For this review, take the finished solid that the model builds, in its own axes (mm). A direction names the side the tool comes from. Give positions to 0.01 mm unless a question says otherwise; leave off trailing zeros. Order: outer loops, then holes, each group sorted by start corner. A loop starts at its lowest first (then second) coordinate and runs counter-clockwise, first axis right, second up.
from build123d import *

# Parameters (mm, degrees)
SKETCH_1_R          = 1.6
SKETCH_1_R_2        = 30
SKETCH_1_R_3        = 2.1
EXTRUDE_1_DEPTH     = 2.5
SKETCH_2_W          = 20
SKETCH_2_H          = 5
EXTRUDE_2_DEPTH     = 5
CUT_EXTRUDE_1_DEPTH = 97.176920308
FILLET_1_R          = 5


with BuildPart() as part:
    # 草图1 → 凸台-拉伸1 (new, symmetric)
    with BuildSketch(Plane(origin=(0, 0, 0), x_dir=(1, 0, 0), z_dir=(0, 1, 0))):
        with BuildLine():
            Line((-60, 0), (-60, -70))
            Line((-60, -70), (60, -70))
            Line((60, -70), (60, 0))
            ThreePointArc((60, 0), (42.426406871, 42.426406871), (0, 60))
            ThreePointArc((0, 60), (-42.426406871, 42.426406871), (-60, 0))
        make_face()
        with Locations(Location((-37.5, 0, 0), (0, 0, 270))):
            Circle(SKETCH_1_R, mode=Mode.SUBTRACT)
        with Locations(Location((-40, -57.62, 0), (0, 0, 270))):
            Circle(SKETCH_1_R, mode=Mode.SUBTRACT)
        with Locations(Location((40, -57.62, 0), (0, 0, 270))):
            Circle(SKETCH_1_R, mode=Mode.SUBTRACT)
        with Locations(Location((0, 0, 0), (0, 0, 270))):
            Circle(SKETCH_1_R_2, mode=Mode.SUBTRACT)
        with Locations(Location((-28.726666617, 24.104535363, 0), (0, 0, 270))):
            Circle(SKETCH_1_R, mode=Mode.SUBTRACT)
        with Locations(Location((-6.511806663, 36.930290738, 0), (0, 0, 270))):
            Circle(SKETCH_1_R, mode=Mode.SUBTRACT)
        with Locations(Location((18.75, 32.475952642, 0), (0, 0, 270))):
            Circle(SKETCH_1_R, mode=Mode.SUBTRACT)
        with Locations(Location((35.238473279, 12.825755375, 0), (0, 0, 270))):
            Circle(SKETCH_1_R, mode=Mode.SUBTRACT)
        with Locations(Location((35.238473279, -12.825755375, 0), (0, 0, 270))):
            Circle(SKETCH_1_R, mode=Mode.SUBTRACT)
        with Locations(Location((18.75, -32.475952642, 0), (0, 0, 270))):
            Circle(SKETCH_1_R, mode=Mode.SUBTRACT)
        with Locations(Location((-6.511806663, -36.930290738, 0), (0, 0, 270))):
            Circle(SKETCH_1_R, mode=Mode.SUBTRACT)
        with Locations(Location((-28.726666617, -24.104535363, 0), (0, 0, 270))):
            Circle(SKETCH_1_R, mode=Mode.SUBTRACT)
        with Locations(Location((-11, -65, 0), (0, 0, 270))):
            Circle(SKETCH_1_R_3, mode=Mode.SUBTRACT)
        with Locations(Location((11, -65, 0), (0, 0, 90))):
            Circle(SKETCH_1_R_3, mode=Mode.SUBTRACT)
        with Locations(Location((40, -47.62, 0), (0, 0, 270))):
            Circle(SKETCH_1_R_3, mode=Mode.SUBTRACT)
        with Locations(Location((40, -37.62, 0), (0, 0, 270))):
            Circle(SKETCH_1_R_3, mode=Mode.SUBTRACT)
        with Locations(Location((40, -27.62, 0), (0, 0, 270))):
            Circle(SKETCH_1_R_3, mode=Mode.SUBTRACT)
        with Locations(Location((0, -54, 0), (0, 0, 270))):
            Circle(SKETCH_1_R, mode=Mode.SUBTRACT)
        with Locations(Location((8.488193337, 40, 0), (0, 0, 270))):
            Circle(SKETCH_1_R, mode=Mode.SUBTRACT)
        with Locations(Location((-1.511806663, 40.862744239, 0), (0, 0, 270))):
            Circle(SKETCH_1_R, mode=Mode.SUBTRACT)
        with Locations(Location((-11.420717282, 39.263426275, 0), (0, 0, 270))):
            Circle(SKETCH_1_R, mode=Mode.SUBTRACT)
    extrude(amount=EXTRUDE_1_DEPTH, both=True)

    # 草图2 → 凸台-拉伸2 (add)
    with BuildSketch(Plane.XY.offset(70)):
        with Locations((40, 0)):
            Rectangle(SKETCH_2_W, SKETCH_2_H)
        with Locations((-40, 0)):
            Rectangle(SKETCH_2_W, SKETCH_2_H)
    extrude(amount=EXTRUDE_2_DEPTH)

    # 草图3 → 切除-拉伸1 (cut, through all)
    with BuildSketch(Plane(origin=(0, 2.5, 0), x_dir=(1, 0, 0), z_dir=(0, 1, 0))):
        with BuildLine():
            ThreePointArc((41.406951107, -17.62), (0, 45), (-41.406951107, -17.62))
            Line((-41.406951107, -17.62), (-60, -70))
            Line((-60, -70), (-60, 0))
            ThreePointArc((-60, 0), (0, 60), (60, 0))
            Line((60, 0), (60, -70))
            Line((60, -70), (41.406951107, -17.62))
        make_face()
    extrude(amount=-CUT_EXTRUDE_1_DEPTH, mode=Mode.SUBTRACT)

    # 圆角1
    fillet_1_edges = [part.edges().sort_by_distance(p)[0] for p in [
        (60, 0, 70),
        (-60, 0, 70),
    ]]
    fillet(fillet_1_edges, radius=FILLET_1_R)


solid = part.part
1) We need section A-A on z = 0. Give the boundary of the cut face in (x, y), then the cut area to 3 significant figures.
Answer sheet:
outline: (-45, -2.5) - (-39.1, -2.5) - (-39.1, 2.5) - (-45, 2.5) - close; (-35.9, -2.5) - (-30, -2.5) - (-30, 2.5) - (-35.9, 2.5) - close; (30, -2.5) - (45, -2.5) - (45, 2.5) - (30, 2.5) - close
area: 134 mm2
2) We need section D-D on z = 43. Give the boundary of the cut face in (x, y).
Answer sheet:
outline: (-50.42, -2.5) - (50.42, -2.5) - (50.42, 2.5) - (-50.42, 2.5) - close
3) Draft analysis for pull direction X (two halves, no side actions). For faces 4 (the face through (1.243, 0.035, -44.983)), 5 (the face through (-1, -2.5, 41)), 6 (the face through (-1.031, -0.035, -39.337)), state which applies: +X half, -X half, draft (parallel to the pull), parting line (faces both ways), or undercut.
Answer sheet:
face 4: parting line
face 5: draft
face 6: undercut
4) To check wall thickness, follow line 1 (X direction, y = -1.15, z = 0); line 2 (X direction, y = 1.45, z = -40); line 3 (X direction, y = 1.15, z = 36). State the ranges of each line that lie inside material, in increasing order.
Answer sheet:
line 1: x = -45 to -39.1, -35.9 to -30, 30 to 45
line 2: x = -20.62 to -12.84, -10 to -2.86, -0.16 to 6.89, 10.09 to 20.62
line 3: x = -47.93 to -7.81, -5.21 to 38.66, 41.34 to 47.93
5) We need section C-C on z = 27.62. Give the boundary of the cut face in (x, y), then the cut area to 3 significant figures.
Answer sheet:
outline: (-44.96, -2.5) - (-11.71, -2.5) - (-11.71, 2.5) - (-44.96, 2.5) - close; (11.71, -2.5) - (37.9, -2.5) - (37.9, 2.5) - (11.71, 2.5) - close; (42.1, -2.5) - (44.96, -2.5) - (44.96, 2.5) - (42.1, 2.5) - close
area: 311 mm2
6) Clearance check with flat-ended pins moving along their axes: pin 1 (1.5 mm diameter, centred on y = 0, z = 72, fed in from -X); pin 2 (4 mm diameter, centred on x = -28.73, z = 24.1, fed in from -Y); pin 3 (1 mm diameter, centred on y = -0.5, z = 37, fed in from -X); pin 4 (2 mm diameter, centred on y = 0.5, z = 9, fed in from +X). State where each tip first meets the part, or that it passes through.
Answer sheet:
pin 1: stops at x = -50
pin 2: stops at y = -2.5
pin 3: stops at x = -48.46
pin 4: stops at x = 44.28
7) Tool access review of faces 1 (the face through (-50, 0, 72)), 2 (the face through (-30, 0, 72)), 3 (the face through (49.63, 0.04, 40.79)): name each direction out of +Z, -Z, +X, -X, +Y, -Y from which nothing blocks a thin tool from reaching the whole face with its end or side.
Answer sheet:
face 1: +Z, -X, +Y, -Y
face 2: +Z, +Y, -Y
face 3: +X, +Y, -Y
8) We need section B-B on y = -1.5. Count the separate pieces of the cut face and the enclosed holes in it, then the cut area to 3 significant figures.
Answer sheet:
separate pieces: 1
enclosed holes: 21
area: 7,200 mm2
